```python
from build123d import *

# Parameters (mm, degrees)
BOSS_EXTRUDE1_DEPTH     = 9
SKETCH1_3_R             = 25
SKETCH1_3_R_2           = 12.5
BOSS_EXTRUDE2_DEPTH     = 23
SKETCH1_5_R             = 28
SKETCH1_5_R_2           = 16
BOSS_EXTRUDE3_DEPTH     = 35
BOSS_EXTRUDE4_DEPTH     = 31
BOSS_EXTRUDE5_DEPTH     = 21
SKETCH1_8_R             = 18
SKETCH1_8_R_2           = 7.5
BOSS_EXTRUDE6_DEPTH     = 24
SKETCH2_W               = 34
SKETCH2_H               = 56
CUT_EXTRUDE1_DEPTH      = 104
CUT_EXTRUDE1_DEPTH_BACK = 29
SKETCH3_W               = 18
SKETCH3_H               = 36
CUT_EXTRUDE2_DEPTH      = 1
CUT_EXTRUDE2_DEPTH_BACK = 164


with BuildPart() as part:
    # Sketch1 → Boss-Extrude1 (new body, symmetric)
    with BuildSketch(Plane(origin=(0, 0, 0), x_dir=(0, 0, -1), z_dir=(1, 0, 0))):
        with BuildLine():
            ThreePointArc((25, 110), (-17.67766953, 92.32233047), (0, 135))
            Line((0, 135), (-55, 135))
            Line((-55, 135), (-55, 99))
            Line((-55, 99), (-25, 99))
            Line((-25, 99), (-25, 40))
            Line((-25, 40), (25, 40))
            Line((25, 40), (25, 110))
        make_face()
    extrude(amount=BOSS_EXTRUDE1_DEPTH, both=True)

    # Sketch1<3> → Boss-Extrude2 (add, symmetric)
    with BuildSketch(Plane(origin=(0, 0, 0), x_dir=(0, 0, -1), z_dir=(1, 0, 0))):
        with Locations((0, 110)):
            Circle(SKETCH1_3_R)
        with Locations((0, 110)):
            Circle(SKETCH1_3_R_2, mode=Mode.SUBTRACT)
    extrude(amount=BOSS_EXTRUDE2_DEPTH, both=True)



with BuildPart() as body_2:
    # Sketch1<5> → Boss-Extrude3 (new body, symmetric)
    with BuildSketch(Plane(origin=(0, 0, 0), x_dir=(0, 0, -1), z_dir=(1, 0, 0))):
        Circle(SKETCH1_5_R)
        Circle(SKETCH1_5_R_2, mode=Mode.SUBTRACT)
    extrude(amount=BOSS_EXTRUDE3_DEPTH, both=True)


with BuildPart() as part_1:
    add(part.part)

    add(body_2.part)  # Boss-Extrude4 merges body 2
    # Sketch1<6> → Boss-Extrude4 (add, symmetric)
    with BuildSketch(Plane(origin=(0, 0, 0), x_dir=(0, 0, -1), z_dir=(1, 0, 0))):
        with BuildLine():
            Line((25, 40), (-25, 40))
            Line((-25, 40), (-25, 12.609520213))
            ThreePointArc((-25, 12.609520213), (0, 28), (25, 12.609520213))
            Line((25, 12.609520213), (25, 40))
        make_face()
    extrude(amount=BOSS_EXTRUDE4_DEPTH, both=True)

    # Sketch1<7> → Boss-Extrude5 (add, symmetric)
    with BuildSketch(Plane(origin=(0, 0, 0), x_dir=(0, 0, -1), z_dir=(1, 0, 0))):
        with BuildLine():
            Line((-85, 99), (-55, 99))
            Line((-55, 99), (-55, 135))
            Line((-55, 135), (-85, 135))
            ThreePointArc((-85, 135), (-72.272077939, 129.727922061), (-67, 117))
            ThreePointArc((-67, 117), (-72.272077939, 104.272077939), (-85, 99))
        make_face()
    extrude(amount=BOSS_EXTRUDE5_DEPTH, both=True)

    # Sketch1<8> → Boss-Extrude6 (add, symmetric)
    with BuildSketch(Plane(origin=(0, 0, 0), x_dir=(0, 0, -1), z_dir=(1, 0, 0))):
        with Locations((-85, 117)):
            Circle(SKETCH1_8_R)
        with Locations((-85, 117)):
            Circle(SKETCH1_8_R_2, mode=Mode.SUBTRACT)
    extrude(amount=BOSS_EXTRUDE6_DEPTH, both=True)

    # Sketch2 → Cut-Extrude1 (cut, two sides)
    with BuildSketch(Plane.XY) as cut_extrude1_sk:
        Rectangle(SKETCH2_W, SKETCH2_H)
    extrude(amount=CUT_EXTRUDE1_DEPTH, mode=Mode.SUBTRACT)
    extrude(cut_extrude1_sk.sketch, amount=-CUT_EXTRUDE1_DEPTH_BACK, mode=Mode.SUBTRACT)

    # Sketch3 → Cut-Extrude2 (cut, two sides)
    with BuildSketch(Plane(origin=(0, 135, 0), x_dir=(1, 0, 0), z_dir=(0, 1, 0))) as cut_extrude2_sk:
        with Locations((0, -85)):
            Rectangle(SKETCH3_W, SKETCH3_H)
    extrude(amount=CUT_EXTRUDE2_DEPTH, mode=Mode.SUBTRACT)
    extrude(cut_extrude2_sk.sketch, amount=-CUT_EXTRUDE2_DEPTH_BACK, mode=Mode.SUBTRACT)


solid = part_1.part
```
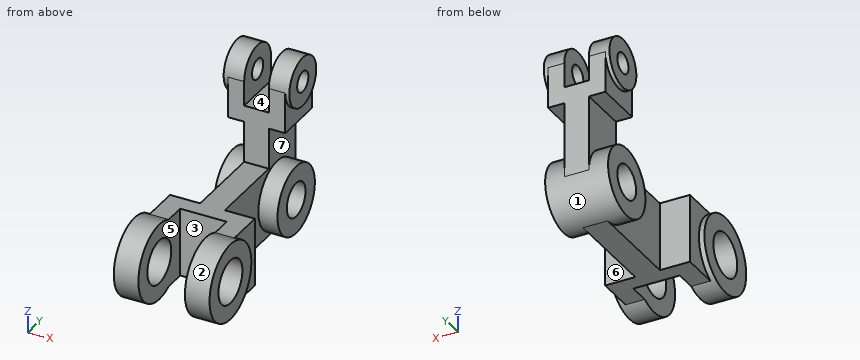
The listing builds one solid part. Answer for the finished solid, in the listing's coordinates (mm). Face numbers are marked on the shaded views. A direction names the side the tool comes from. Round coordinates to 2 decimals unless told otherwise and drop trailing zeros. Order: outer loops, then holes, each group sorted by start corner. A loop starts at its lowest first (then second) coordinate and runs counter-clockwise, first axis right, second up. Notation, with made-up numbers: (61.5, 42.25) - (96.5, 42.25) arc R12 ccw to (96.5, 64.25) - close; hole circle Ø11 at (70, 81.25). An arc over 180 degrees is marked (long way). Put each result on its own line as item: value. Start each with the question number.
(1) For the marked faces 4, 5, 6 and 7, determine the directions among +Z, -Z, +X, -X, +Y, -Y from which every point of the face is accessible in a straight line to the end or side of a thin tool.
(2) Find section A-A (x = -26.5). Give the vertices of the cut face in (y, z), plus the area to 3 significant figures.
(3) Find section C-C (z = 88.5). Give the vertices of the cut face in (x, y), plus the area to 3 significant figures.
(4) Given P1, Ø15, axis at y = 99.5, z = -5, coming from the +X side; P2, Ø14.5, axis at x = 0, y = 109, coming from the +Z side; P3, Ø3, axis at y = 27, z = 17, coming from the -X side, each flat-ended and moving along its own axis, determine where each tip first touches the part or whether it passes through.
(5) Determine the mould class of the marked faces 1, 2 and 3 for opening direction Z: released by +Z, released by -Z, zero draft, split by the parting line, or undercut.
(6) Straight lines are drawn through the part: probe 1 along Y at (x, z) = (-13, 0); probe 2 along Y at (x, z) = (20.75, 85); probe 3 along X at (y, z) = (9, 19). For each, find the intervals that lie inside material, in ascending order. Write a range as from..to.
(7) Find section B-B (y = 0). Give the vertices of the cut face in (x, z), plus the area to 3 significant figures.
(8) Find section D-D (x = -1.5). Give the vertices of the cut face in (y, z), plus the area to 3 significant figures.
Reply:
1. face 4: +Z, +Y, -Y
1. face 5: +Z, -Z, -Y
1. face 6: +Z, -Z, +X
1. face 7: +X
2. outline: (12.61, -25) - (40, -25) - (40, 25) - (12.61, 25) arc R28 ccw (long way) to start; hole circle Ø32 at (0, 0)
2. area: 2,480 mm^2
3. outline: (-24, 99.34) - (-9, 99.34) - (-9, 110.37) - (-24, 110.37) - close; (-24, 123.63) - (-9, 123.63) - (-9, 134.66) - (-24, 134.66) - close; (9, 99.34) - (24, 99.34) - (24, 110.37) - (9, 110.37) - close; (9, 123.63) - (24, 123.63) - (24, 134.66) - (9, 134.66) - close
3. area: 661 mm^2
4. P1: x = 23
4. P2: z = 67
4. P3: x = -31
5. face 1: undercut
5. face 2: split by the parting line
5. face 3: zero draft
6. probe 1: 28..40, 85..97.5, 122.5..135
6. probe 2: 99..109.5, 124.5..135
6. probe 3: -35..-17, 17..35
7. outline: (-35, -28) - (-17, -28) - (-17, -16) - (-35, -16) - close; (-35, 16) - (-17, 16) - (-17, 28) - (-35, 28) - close; (17, -28) - (35, -28) - (35, -16) - (17, -16) - close; (17, 16) - (35, 16) - (35, 28) - (17, 28) - close
7. area: 864 mm^2
8. outline: (28, -25) - (110, -25) arc R25 ccw to (135, 0) - (135, 67) - (99, 67) - (99, 25) - (28, 25) - close; hole circle Ø25 at (110, 0)
8. area: 6,240 mm^2
